Autodesk Inventor part; units mm, degrees
ref_plane "YZ Plane" through (0, 0, 0) normal (1, 0, 0) x (0, 1, 0)
ref_plane "XZ Plane" through (0, 0, 0) normal (0, 1, 0) x (-1, 0, 0)
ref_plane "XY Plane" through (0, 0, 0) normal (0, 0, 1) x (1, 0, 0)
sketch "스케치1" plane through (0, 0, 0) normal (0, 1, 0) x (-1, 0, 0)
  circle A0 centre (0, 0) radius 1.5
  dimension "d0" = 3
extrude "돌출1" add sketch "스케치1" along normal blind 50
sketch "스케치2" plane through (0, 0, 0) normal (0, 1, 0) x (-1, 0, 0)
  arc A0 (0, 3) -> (0, -3) centre (0, 0) ccw
  line L0 (0, 3) -> (0, -3)
  line L1 (0, -7) -> (0, 7)
  dimension "d3" = 6
revolve "회전1" add sketch "스케치2" angle 360 about axis through (0, 0, -10) along (0, 0, 1)
sketch "스케치3" plane through (0, 0, 0) normal (0, 0, 1) x (1, 0, 0)
  circle A0 centre (0, 0) radius 1.5
  dimension "d5" = 3
extrude "돌출2" add sketch "스케치3" along normal blind 50
sketch "스케치4" plane through (0, 0, 0) normal (1, 0, 0) x (0, 1, 0)
  circle A0 centre (0, 0) radius 1.5
  dimension "d8" = 3
extrude "돌출3" add sketch "스케치4" against normal blind 50
properties part number "arrows2"
Here's how the part is built. I have some questions about the finished solid (model axes, mm). A direction names the side the tool comes from. Coordinates: 2 decimals unless noted, no trailing zeros. Loops run counter-clockwise (first coordinate to the right, second up) from the corner with the lowest first, then second, coordinate; pieces in that order, holes last. Notation, with made-up numbers: (17, 64.25) - (28, 64.25) arc R6 cw to (28, 70.25) - close; hole circle Ø4 at (-38, 30). An arc over 180 degrees is marked (long way). Answer as CSV lines item,"result".
Q1. For pin 1 (10 mm diameter, centred on y = 32, z = 3, fed in from -X); pin 2 (5 mm diameter, centred on y = 24, z = 2.5, fed in from +X); pin 3 (12 mm diameter, centred on x = -3.5, y = 30.5, fed in from +Z), each with a flat end and sliding along its axis, tell me the tip position at first contact or that it passes through.
Response:
pin 1,"x = -1.5"
pin 2,"x = 1.5"
pin 3,"z = 1.5"
Q2. If we section it at B-B, the plane x = 0: Write out the boundary of the cut face in (y, z), and give its area (3 significant figures).
Response:
outline,"(-1.5, 2.6) arc R3 ccw (long way) to (2.6, -1.5) - (50, -1.5) - (50, 1.5) - (2.6, 1.5) arc R3 ccw to (1.5, 2.6) - (1.5, 50) - (-1.5, 50) - close"
area,"311 mm2"
Q3. If we section it at C-C, the plane y = 32: Write out the boundary of the cut face in (x, z).
Response:
outline,"circle Ø3 at (0, 0)"
Q4. For faces 1 (the face through (-25.97, -1.5, 0.07)), 2 (the face through (1.5, 25.97, -0.07)), 3 (the face through (-1.5, -0.07, 25.97)), which set-ups out of +Z, -Z, +X, -X, +Y, -Y let a thin tool reach every point of the face, with its end or its side?
Response:
face 1,"-X"
face 2,"+Y"
face 3,"+Z"
Q5. If I drill on L1, parallel to X at y = 0, z = 34.5, over which ranges is the centre line in solid material (lowest first)? Write a range as [from, to].
Response:
L1,"[-1.5, 1.5]"
Q6. If we section it at A-A, the plane z = 0: Write out the boundary of the cut face in (x, y), and give its area (3 significant figures).
Response:
outline,"(-50, -1.5) - (-2.6, -1.5) arc R3 ccw (long way) to (1.5, 2.6) - (1.5, 50) - (-1.5, 50) - (-1.5, 2.6) arc R3 ccw to (-2.6, 1.5) - (-50, 1.5) - close"
area,"311 mm2"
